Source: CAD feature listing. Evaluate the final solid. Frame: model axes, mm. A direction names the side the tool comes from. Round coordinates to 2 decimals unless told otherwise and drop trailing zeros. Use CSV: the item, a comma, the result in double quotes. Start each with the question number.
from build123d import *

# Parameters (mm, degrees)
F1_DEPTH = 781.05


with BuildPart() as f1:
    # F0 (on Right) → F1 (new body)
    with BuildSketch(Plane.YZ):
        Polygon((-57.224485, 18.603526), (-49.726797, 7.954637), (-37.909164, 2.481273), (-24.938112, 3.650017), (-14.289223, 11.147705), (-8.815859, 22.965337), (-9.620451, 31.894936), (-11.24866, 31.116622), (-13.236551, 30.457316), (-15.291399, 30.052357), (-15.607873, 30.030512), (-19.835498, 13.723182), (-38.451873, 8.572227), (-52.220918, 22.119002), (-47.373589, 40.816733), (-33.998333, 44.517526), (-34.120155, 45.436821), (-34.1329, 47.531154), (-33.883056, 49.610571), (-33.374561, 51.642276), (-33.354722, 51.693289), (-42.270976, 50.889899), (-52.919864, 43.392211), (-58.393229, 31.574578), align=None)
        Polygon((-17.3808, 29.908133), (-15.607873, 30.030512), (-14.988169, 32.420913), (-28.757215, 45.967688), (-33.998333, 44.517526), (-33.845021, 43.3606), (-33.311836, 41.335233), (-32.52901, 39.392663), (-31.508889, 37.563525), (-30.26756, 35.876666), (-28.824599, 34.358687), (-27.202763, 33.033529), (-25.42763, 31.922091), (-23.527194, 31.041899), (-21.531426, 30.406836), (-19.471801, 30.026917), align=None)
        Polygon((-32.615436, 53.59423), (-33.354722, 51.693289), (-29.299923, 52.058643), (-17.482291, 46.585278), (-9.984603, 35.936389), (-9.620451, 31.894936), (-9.359077, 32.019878), (-7.597603, 33.152839), (-5.992015, 34.497638), (-4.567636, 36.033066), (-3.346929, 37.734908), (-2.349145, 39.576327), (-1.59002, 41.52828), (-1.081526, 43.559986), (-0.831681, 45.639402), (-0.844426, 47.733735), (-1.119561, 49.809957), (-1.652745, 51.835323), (-2.435571, 53.777893), (-3.455692, 55.607031), (-4.697022, 57.293891), (-6.139982, 58.811869), (-7.761818, 60.137027), (-9.536951, 61.248466), (-11.437388, 62.128657), (-13.433155, 62.76372), (-15.492781, 63.14364), (-17.583781, 63.262424), (-19.673182, 63.118199), (-21.72803, 62.713241), (-23.715921, 62.053935), (-25.605504, 61.150679), (-27.366979, 60.017718), (-28.972566, 58.672919), (-30.396945, 57.137491), (-31.617652, 55.435648), align=None)
        Polygon((-29.299923, 52.058643), (-33.354722, 51.693289), (-33.374561, 51.642276), (-33.883056, 49.610571), (-34.1329, 47.531154), (-34.120155, 45.436821), (-33.998333, 44.517526), (-28.757215, 45.967688), (-14.988169, 32.420913), (-15.607873, 30.030512), (-15.291399, 30.052357), (-13.236551, 30.457316), (-11.24866, 31.116622), (-9.620451, 31.894936), (-9.984603, 35.936389), (-17.482291, 46.585278), align=None)
    extrude(amount=-F1_DEPTH)


solid = f1.part
1. Mould query, pull axis Y, two halves, no side actions, for faces 1 (the flat face through (-781.05, -24, 33)), 2 (the flat face through (-385.06, -40.78, 42.64)), 3 (the flat face through (-385.058, -43.901, 5.256)). Classes: +Y half, -Y half, draft (parallel to the pull), parting line (faces both ways), or undercut.
2. Line query: line 1 along Z through (x, y) = (-374, -40); line 2 along Y through (x, z) = (-554, 23.5); line 3 along Y through (x, z) = (-615.5, 23). Output: solid intervals per line, ascending.
3. Contact query for flat-ended pins moving along their axis: P1, Ø4, axis at y = -10, z = 11.5, coming from the -X side; P2, Ø3, axis at x = -452, z = 52, coming from the +Y side; P3, Ø5, axis at x = -241, z = 53.5, coming from the +Y side; P4, Ø4, axis at x = -85.5, y = -22, coming from the +Z side. Output: stop coordinate, or through.
4. Reachability of faces 4 (the flat face through (-385.058, -31.514, 3.057)), 5 (the flat face through (-385.06, -45.24, 15.25)) from +Z, -Z, +X, -X, +Y, -Y: full face, straight path, thin tool, end or side. Return the list, or none.
Values:
1,face 1,"draft"
1,face 2,"undercut"
1,face 3,"-Y half"
2,line 1,"z = 3.45 to 10.1, 42.86 to 51.09"
2,line 2,"y = -57.67 to -51.86, -17.3 to -8.86"
2,line 3,"y = -57.62 to -51.99, -17.43 to -8.82"
3,P1,"passes through"
3,P2,"stops at y = -1.3"
3,P3,"stops at y = -1.43"
3,P4,"stops at z = 63.05"
4,face 4,"-Z, +X, -X, +Y"
4,face 5,"+X, -X"
